Input: dimensioned drawing with shaded views. Units: mm. Origin: part minimum x, y, z. Coordinates: 2 decimals unless noted, no trailing zeros. Order: outer loops, then holes, each group sorted by start corner. A loop starts at its lowest first (then second) coordinate and runs counter-clockwise, first axis right, second up. Notation, with made-up numbers: (27, 0) -> (75, 0) arc R9 cw to (75, 13) -> close; hole circle Ø2 at (65.25, -5.75). An arc over 180 degrees is marked (long way). Answer as CSV lines item,"result".
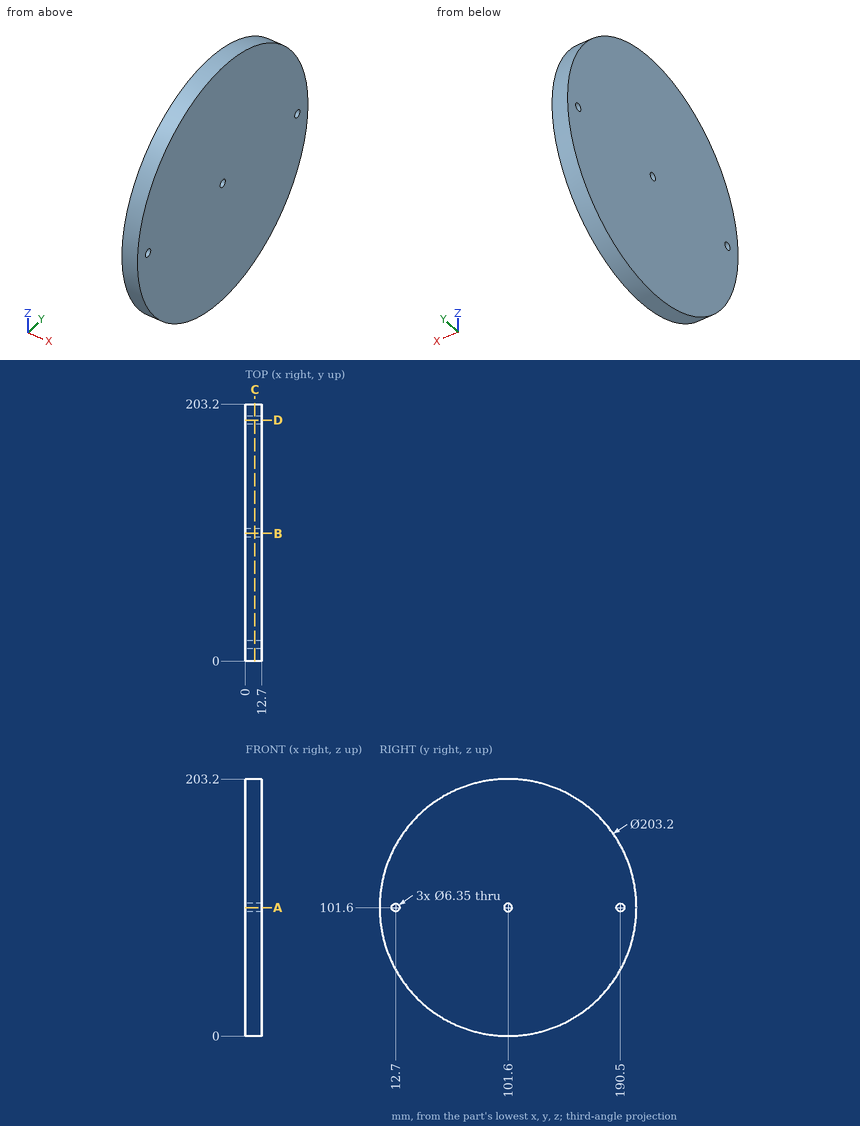
1. Contact query for flat-ended pins moving along their axis: pin 1 (1 mm diameter, centred on x = 2.5, y = 178, fed in from -Z); pin 2 (2 mm diameter, centred on x = 8.5, y = 115.5, fed in from +Z); pin 3 (1 mm diameter, centred on x = 3.5, y = 68, fed in from +Z); pin 4 (4 mm diameter, centred on y = 190.5, z = 101.6, fed in from +X). Output: stop coordinate, or through.
Findings:
pin 1,"stops at z = 34.06"
pin 2,"stops at z = 202.38"
pin 3,"stops at z = 197.66"
pin 4,"passes through"
2. Cut plane B-B (y = 101). Return the cut outline in (x, z), plus the area to 3 significant figures.
Findings:
outline,"(0, 0) -> (12.7, 0) -> (12.7, 98.48) -> (0, 98.48) -> close; (0, 104.72) -> (12.7, 104.72) -> (12.7, 203.2) -> (0, 203.2) -> close"
area,"2,500 mm2"
3. Ray query, line 1 along Z through (x, y) = (8, 101.6) (3 decimals); line 2 along Z through (x, y) = (8.25, 12.7) (3 decimals); line 3 along Z through (x, y) = (7, 85.5). Return the intervals inside material, ascending.
Findings:
line 1,"z = 0 to 98.425, 104.775 to 203.2"
line 2,"z = 52.413 to 98.425, 104.775 to 150.787"
line 3,"z = 1.28 to 201.92"
4. Cut plane A-A (z = 101.6). Return the cut outline in (x, y) (3 decimals).
Findings:
outline,"(0, 0) -> (12.7, 0) -> (12.7, 9.525) -> (0, 9.525) -> close; (0, 15.875) -> (12.7, 15.875) -> (12.7, 98.425) -> (0, 98.425) -> close; (0, 104.775) -> (12.7, 104.775) -> (12.7, 187.325) -> (0, 187.325) -> close; (0, 193.675) -> (12.7, 193.675) -> (12.7, 203.2) -> (0, 203.2) -> close"
5. Cut plane D-D (y = 190.5). Return the cut outline in (x, z) (3 decimals), plus the area to 3 significant figures.
Findings:
outline,"(0, 52.413) -> (12.7, 52.413) -> (12.7, 98.425) -> (0, 98.425) -> close; (0, 104.775) -> (12.7, 104.775) -> (12.7, 150.787) -> (0, 150.787) -> close"
area,"1,170 mm2"
6. Cut plane C-C (x = 7.5). Return the cut outline in (y, z) (3 decimals), plus the area to 3 significant figures.
Findings:
outline,"circle Ø203.2 at (101.6, 101.6); hole circle Ø6.35 at (12.7, 101.6); hole circle Ø6.35 at (101.6, 101.6); hole circle Ø6.35 at (190.5, 101.6)"
area,"32,300 mm2"
